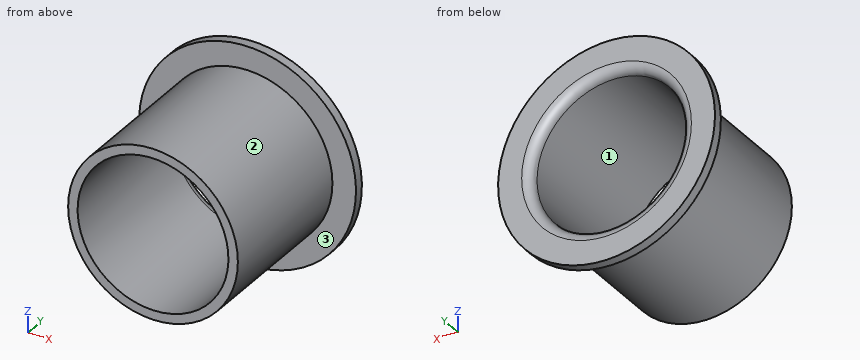
```python
from build123d import *


with BuildPart() as part:
    # 草图1 → 旋转-薄壁1 (revolve)
    with BuildSketch(Plane(origin=(0, 0, 0), x_dir=(0, 0, -1), z_dir=(1, 0, 0))):
        with BuildLine():
            Line((8, 0.906546657), (8, 16.906546657))
            ThreePointArc((8, 16.906546657), (8.292893219, 17.613653438), (9, 17.906546657))
            Line((9, 17.906546657), (11.5, 17.906546657))
            Line((11.5, 17.906546657), (11.5, 16.906546657))
            Line((11.5, 16.906546657), (9, 16.906546657))
            Line((9, 16.906546657), (9, 0.906546657))
            Line((9, 0.906546657), (8, 0.906546657))
        make_face()
    revolve(axis=Axis((0, 0, 0), (0, 1, 0)))


solid = part.part
```
Read the model definition and answer for the solid it produces. Units are mm, in the model's axes. Face numbers are marked on the shaded views. Round coordinates to 2 decimals unless told otherwise and drop trailing zeros. Write each loop counter-clockwise with the first axis right and the second up, starting at its lowest first coordinate (ties: lowest second). Pieces come first, ordered by that corner, then holes. Notation, with made-up numbers: (-6, -14.5) - (44, -14.5) arc R28 cw to (44, 12.5) - close; hole circle Ø3 at (13.25, 72). An arc over 180 degrees is marked (long way). One line per item, written item: value.
Q1. For a pull along Z with two mould halves and no side action, classify the marked faces 1, 2 and 3 as pulls with the +Z half, pulls with the -Z half, needs draft (parallel to the pull), parting line crosses it, or undercut.
The answers:
face 1: undercut
face 2: parting line crosses it
face 3: needs draft
Q2. Straight lines are drawn through the part: line 1 (Z direction, x = 0, y = 12); line 2 (X direction, y = 7.75, z = 3.25). For each, find the intervals that lie inside material, in ascending order. Write a range as from..to.
The answers:
line 1: z = -9..-8, 8..9
line 2: x = -8.39..-7.31, 7.31..8.39
Q3. Find section B-B (x = 0). Determine the outline of the cut face in (y, z), and give its area (3 significant figures).
The answers:
outline: (0.91, -9) - (16.91, -9) - (16.91, -11.5) - (17.91, -11.5) - (17.91, -9) arc R1 ccw to (16.91, -8) - (0.91, -8) - close; (0.91, 8) - (16.91, 8) arc R1 ccw to (17.91, 9) - (17.91, 11.5) - (16.91, 11.5) - (16.91, 9) - (0.91, 9) - close
area: 38.6 mm2
Q4. Find section A-A (z = 0). Determine the outline of the cut face in (x, y), and give its area (3 significant figures).
The answers:
outline: (-11.5, 16.91) - (-9, 16.91) - (-9, 0.91) - (-8, 0.91) - (-8, 16.91) arc R1 ccw to (-9, 17.91) - (-11.5, 17.91) - close; (8, 0.91) - (9, 0.91) - (9, 16.91) - (11.5, 16.91) - (11.5, 17.91) - (9, 17.91) arc R1 ccw to (8, 16.91) - close
area: 38.6 mm2
Q5. Find section C-C (y = 12). Determine the outline of the cut face in (x, z), and give its area (3 significant figures).
The answers:
outline: circle Ø18 at (0, 0); hole circle Ø16 at (0, 0)
area: 53.4 mm2
Q6. Each of these flat-tipped pins is pushed along its axis until it touches: P1, Ø6, axis at x = -4, z = -3.5, coming from the -Y side; P2, Ø1, axis at y = 3, z = -6, coming from the -X side; P3, Ø3, axis at x = 3.5, y = 3, coming from the +Z side; P4, Ø1.5, axis at x = -9, y = 14, coming from the -Z side. Where does it stop, or does it pass through?
The answers:
P1: stops at y = 0.91
P2: stops at x = -7.12
P3: stops at z = 8.77
P4: stops at z = -3.6
